Read the model definition and answer for the solid it produces. Units are mm, in the model's axes. A direction names the side the tool comes from. Give positions to 0.01 mm unless a question says otherwise; leave off trailing zeros. Write each loop counter-clockwise with the first axis right and the second up, starting at its lowest first coordinate (ties: lowest second). Pieces come first, ordered by that corner, then holes.
```python
from build123d import *

# Parameters (mm, degrees)
BOSS_EXTRUDE1_DEPTH = 10
CUT_EXTRUDE3_REACH  = 12
SKETCH2_R           = 2.05
SKETCH5_R           = 4
CUT_EXTRUDE4_DEPTH  = 5


with BuildPart() as part:
    # Sketch1 → Boss-Extrude1 (new body)
    with BuildSketch(Plane(origin=(0, 0, 0), x_dir=(1, 0, 0), z_dir=(0, 1, 0))):
        Polygon((-41.160131748, 19.796063365), (-41.160131748, -65.203936635), (43.839868252, -65.203936635), (43.839868252, -9.902421445), (14.141383442, 19.796063365), align=None)
    extrude(amount=BOSS_EXTRUDE1_DEPTH)

    # Sketch2 → Cut-Extrude3 (cut, up to next)
    with BuildSketch(Plane(origin=(0, 10, 0), x_dir=(1, 0, 0), z_dir=(0, 1, 0)), mode=Mode.PRIVATE) as cut_extrude3_sk1:
        with Locations((37.839868252, -12.387702819)):
            Circle(SKETCH2_R)
    cut_extrude3_tool1 = extrude(cut_extrude3_sk1.sketch, amount=-CUT_EXTRUDE3_REACH, mode=Mode.PRIVATE) & part.part
    add(cut_extrude3_tool1.solids().sort_by_distance((37.839868, 10, 12.387703))[0], mode=Mode.SUBTRACT)
    # Sketch2 → Cut-Extrude3 (cut, up to next)
    with BuildSketch(Plane(origin=(0, 10, 0), x_dir=(1, 0, 0), z_dir=(0, 1, 0)), mode=Mode.PRIVATE) as cut_extrude3_sk2:
        with Locations((37.839868252, -59.203936635)):
            Circle(SKETCH2_R)
    cut_extrude3_tool2 = extrude(cut_extrude3_sk2.sketch, amount=-CUT_EXTRUDE3_REACH, mode=Mode.PRIVATE) & part.part
    add(cut_extrude3_tool2.solids().sort_by_distance((37.839868, 10, 59.203937))[0], mode=Mode.SUBTRACT)
    # Sketch2 → Cut-Extrude3 (cut, up to next)
    with BuildSketch(Plane(origin=(0, 10, 0), x_dir=(1, 0, 0), z_dir=(0, 1, 0)), mode=Mode.PRIVATE) as cut_extrude3_sk3:
        with Locations((-35.160131748, -59.203936635)):
            Circle(SKETCH2_R)
    cut_extrude3_tool3 = extrude(cut_extrude3_sk3.sketch, amount=-CUT_EXTRUDE3_REACH, mode=Mode.PRIVATE) & part.part
    add(cut_extrude3_tool3.solids().sort_by_distance((-35.160132, 10, 59.203937))[0], mode=Mode.SUBTRACT)
    # Sketch2 → Cut-Extrude3 (cut, up to next)
    with BuildSketch(Plane(origin=(0, 10, 0), x_dir=(1, 0, 0), z_dir=(0, 1, 0)), mode=Mode.PRIVATE) as cut_extrude3_sk4:
        with Locations((-35.160131748, 13.796063365)):
            Circle(SKETCH2_R)
    cut_extrude3_tool4 = extrude(cut_extrude3_sk4.sketch, amount=-CUT_EXTRUDE3_REACH, mode=Mode.PRIVATE) & part.part
    add(cut_extrude3_tool4.solids().sort_by_distance((-35.160132, 10, -13.796063))[0], mode=Mode.SUBTRACT)
    # Sketch2 → Cut-Extrude3 (cut, up to next)
    with BuildSketch(Plane(origin=(0, 10, 0), x_dir=(1, 0, 0), z_dir=(0, 1, 0)), mode=Mode.PRIVATE) as cut_extrude3_sk5:
        with Locations((11.656102068, 13.796063365)):
            Circle(SKETCH2_R)
    cut_extrude3_tool5 = extrude(cut_extrude3_sk5.sketch, amount=-CUT_EXTRUDE3_REACH, mode=Mode.PRIVATE) & part.part
    add(cut_extrude3_tool5.solids().sort_by_distance((11.656102, 10, -13.796063))[0], mode=Mode.SUBTRACT)

    # Sketch5 → Cut-Extrude4 (cut)
    with BuildSketch(Plane.XZ):
        with Locations((37.839868252, 59.203936635)):
            Circle(SKETCH5_R)
        with Locations((37.839868252, 12.387702819)):
            Circle(SKETCH5_R)
        with Locations((11.656102068, -13.796063365)):
            Circle(SKETCH5_R)
        with Locations((-35.160131748, -13.796063365)):
            Circle(SKETCH5_R)
        with Locations((-35.160131748, 59.203936635)):
            Circle(SKETCH5_R)
    extrude(amount=-CUT_EXTRUDE4_DEPTH, mode=Mode.SUBTRACT)


solid = part.part
```
Item 1: Section C-C (x = 20.5) is taken. Write down the section's boundary in (y, z).
Result set:
outline: (0, -13.44) - (10, -13.44) - (10, 65.2) - (0, 65.2) - close
Item 2: Section B-B (y = 2.5) is taken. Write down the section's boundary in (x, z), and give its area (3 significant figures).
Result set:
outline: (-41.16, -19.8) - (14.14, -19.8) - (43.84, 9.9) - (43.84, 65.2) - (-41.16, 65.2) - close; hole circle Ø8 at (-35.16, -13.8); hole circle Ø8 at (-35.16, 59.2); hole circle Ø8 at (11.66, -13.8); hole circle Ø8 at (37.84, 12.39); hole circle Ø8 at (37.84, 59.2)
area: 6,530 mm2
Item 3: Determine the mould class of faces 3 (the flat face through (1, 0, 22)), 4 (the flat face through (-33, 5, -16)), 5 (the cylindrical face through (-35.43, 7.54, 57.17)), 6 (the flat face through (-41.16, 5, 22)) for opening direction X: pulls with the +X half, pulls with the -X half, needs draft (parallel to the pull), parting line crosses it, or undercut.
Result set:
face 3: needs draft
face 4: undercut
face 5: undercut
face 6: pulls with the -X half
Item 4: Which of the six approach directions +Z, -Z, +X, -X, +Y, -Y give full straight-line access (tool end or side, diameter ignored) to faces 1 (the flat face through (40, 5, 11)), 2 (the cylindrical face through (-34.21, 7.54, -11.98))?
Result set:
face 1: -Y
face 2: +Y, -Y
Item 5: Find the intervals of material crossed by line 1 along Z through (x, y) = (39.5, 4); line 2 along Z through (x, y) = (-36.5, 1); line 3 along X through (y, z) = (1, -13.5), in increasing order.
Result set:
line 1: z = 5.56 to 8.75, 16.03 to 55.56, 62.84 to 65.2
line 2: z = -19.8 to -17.56, -10.03 to 55.44, 62.97 to 65.2
line 3: x = -41.16 to -39.15, -31.17 to 7.67, 15.65 to 20.44
Item 6: Section A-A (y = 8) is taken. Write down the section's boundary in (x, z), and give its area (3 significant figures).
Result set:
outline: (-41.16, -19.8) - (14.14, -19.8) - (43.84, 9.9) - (43.84, 65.2) - (-41.16, 65.2) - close; hole circle Ø4.1 at (-35.16, -13.8); hole circle Ø4.1 at (-35.16, 59.2); hole circle Ø4.1 at (11.66, -13.8); hole circle Ø4.1 at (37.84, 12.39); hole circle Ø4.1 at (37.84, 59.2)
area: 6,720 mm2
Item 7: Each of these flat-tipped pins is pushed along its axis until it touches: pin 1 Ø6.5 at (x, z) = (-35.16, 59.2) entering from +Y; pin 2 Ø2.5 at (x, z) = (37.84, 12.39) entering from -Y; pin 3 Ø4 at (x, z) = (10, -14) entering from -Y. Where does it stop, or does it pass through?
Result set:
pin 1: stops at y = 10
pin 2: passes through
pin 3: stops at y = 5
